from build123d import *

# Parameters (mm, degrees)
SKETCH1_W            = 145.4
SKETCH1_H            = 52.4
BOSS_EXTRUDE1_DEPTH  = 27.2
SKETCH2_W            = 140.4
SKETCH2_H            = 47.4
CUT_EXTRUDE1_DEPTH   = 25.2
SKETCH3_W            = 46.4
SKETCH3_H            = 25.2
CUT_EXTRUDE2_DEPTH   = 25.2
SKETCH8_W            = 2.5
SKETCH8_H            = 52.4
CUT_EXTRUDE5_DEPTH   = 43
SKETCH9_W            = 44.4
SKETCH9_H            = 17.2
CUT_EXTRUDE6_DEPTH   = 43
SKETCH11_W           = 132.9
SKETCH11_H           = 16.2
CUT_EXTRUDE7_DEPTH   = 59
SKETCH12_W           = 130.4
SKETCH12_H           = 42.4
CUT_EXTRUDE8_DEPTH   = 10
SKETCH16_W           = 12
SKETCH16_H           = 2.5
BOSS_EXTRUDE4_DEPTH  = 8
SKETCH18_W           = 12
SKETCH18_H           = 2.5
BOSS_EXTRUDE6_DEPTH  = 8
SKETCH24_W           = 10
SKETCH24_H           = 5
BOSS_EXTRUDE12_DEPTH = 6.2
SKETCH25_W           = 10
SKETCH25_H           = 5
BOSS_EXTRUDE13_DEPTH = 6.2
SKETCH26_W           = 10
SKETCH26_H           = 5
BOSS_EXTRUDE14_DEPTH = 9.7
SKETCH27_W           = 10
SKETCH27_H           = 9
BOSS_EXTRUDE15_DEPTH = 5
SKETCH28_W           = 10
SKETCH28_H           = 2
BOSS_EXTRUDE16_DEPTH = 42.4
SKETCH29_W           = 10
SKETCH29_H           = 2
BOSS_EXTRUDE17_DEPTH = 42.4
SKETCH30_W           = 12
SKETCH30_H           = 4
BOSS_EXTRUDE18_DEPTH = 10
SKETCH35_W           = 10
SKETCH35_H           = 6
BOSS_EXTRUDE22_DEPTH = 9
SKETCH36_W           = 10
SKETCH36_H           = 6
BOSS_EXTRUDE23_DEPTH = 9
SKETCH37_R           = 1.5
CUT_EXTRUDE10_DEPTH  = 9
SKETCH38_W           = 10
SKETCH38_H           = 2
CUT_EXTRUDE11_DEPTH  = 9
SKETCH39_W           = 10
SKETCH39_H           = 2
CUT_EXTRUDE12_DEPTH  = 9
SKETCH40_W           = 10
SKETCH40_H           = 2
CUT_EXTRUDE13_DEPTH  = 9
FILLET1_R            = 1


with BuildPart() as part:
    # Sketch1 → Boss-Extrude1 (new body)
    with BuildSketch(Plane(origin=(0, 0, 0), x_dir=(1, 0, 0), z_dir=(0, 1, 0))):
        Rectangle(SKETCH1_W, SKETCH1_H)
    extrude(amount=BOSS_EXTRUDE1_DEPTH)

    # Sketch2 → Cut-Extrude1 (cut)
    with BuildSketch(Plane(origin=(0, 27.2, 0), x_dir=(1, 0, 0), z_dir=(0, 1, 0))):
        Rectangle(SKETCH2_W, SKETCH2_H)
    extrude(amount=-CUT_EXTRUDE1_DEPTH, mode=Mode.SUBTRACT)

    # Sketch3 → Cut-Extrude2 (cut)
    with BuildSketch(Plane.ZY.offset(-70.2)):
        with Locations((0.5, 14.6)):
            Rectangle(SKETCH3_W, SKETCH3_H)
    extrude(amount=-CUT_EXTRUDE2_DEPTH, mode=Mode.SUBTRACT)

    # Sketch8 → Cut-Extrude5 (cut)
    with BuildSketch(Plane(origin=(0, 27.2, 0), x_dir=(1, 0, 0), z_dir=(0, 1, 0))):
        with Locations((71.45, 0)):
            Rectangle(SKETCH8_W, SKETCH8_H)
    extrude(amount=-CUT_EXTRUDE5_DEPTH, mode=Mode.SUBTRACT)

    # Sketch9 → Cut-Extrude6 (cut)
    with BuildSketch(Plane.ZY.offset(72.7)):
        with Locations((0, 13.6)):
            Rectangle(SKETCH9_W, SKETCH9_H)
    extrude(amount=-CUT_EXTRUDE6_DEPTH, mode=Mode.SUBTRACT)

    # Sketch11 → Cut-Extrude7 (cut)
    with BuildSketch(Plane(origin=(0, 0, -26.2), x_dir=(-1, 0, 0), z_dir=(0, 0, -1))):
        with Locations((1.25, 13.1)):
            Rectangle(SKETCH11_W, SKETCH11_H)
    extrude(amount=-CUT_EXTRUDE7_DEPTH, mode=Mode.SUBTRACT)

    # Sketch12 → Cut-Extrude8 (cut)
    with BuildSketch(Plane(origin=(0, 0, 0), x_dir=(-1, 0, 0), z_dir=(0, -1, 0))):
        Rectangle(SKETCH12_W, SKETCH12_H)
    extrude(amount=-CUT_EXTRUDE8_DEPTH, mode=Mode.SUBTRACT)

    # Sketch16 → Boss-Extrude4 (add)
    with BuildSketch(Plane(origin=(0, 0, -26.2), x_dir=(-1, 0, 0), z_dir=(0, 0, -1))):
        with Locations((-64.2, 25.95)):
            Rectangle(SKETCH16_W, SKETCH16_H)
    extrude(amount=BOSS_EXTRUDE4_DEPTH)

    # Sketch18 → Boss-Extrude6 (add)
    with BuildSketch(Plane.XY.offset(26.2)):
        with Locations((64.2, 25.95)):
            Rectangle(SKETCH18_W, SKETCH18_H)
    extrude(amount=BOSS_EXTRUDE6_DEPTH)

    # Sketch24 → Boss-Extrude12 (add)
    with BuildSketch(Plane.XY.offset(26.2)):
        with Locations((-40.7, 2.5)):
            Rectangle(SKETCH24_W, SKETCH24_H)
        with Locations((32.2, 2.5)):
            Rectangle(SKETCH24_W, SKETCH24_H)
    extrude(amount=BOSS_EXTRUDE12_DEPTH)

    # Sketch25 → Boss-Extrude13 (add)
    with BuildSketch(Plane(origin=(0, 0, -26.2), x_dir=(-1, 0, 0), z_dir=(0, 0, -1))):
        with Locations((40.7, 2.5)):
            Rectangle(SKETCH25_W, SKETCH25_H)
        with Locations((-32.2, 2.5)):
            Rectangle(SKETCH25_W, SKETCH25_H)
    extrude(amount=BOSS_EXTRUDE13_DEPTH)

    # Sketch26 → Boss-Extrude14 (add)
    with BuildSketch(Plane(origin=(0, 0, 0), x_dir=(-1, 0, 0), z_dir=(0, -1, 0))):
        with Locations((40.7, 29.9)):
            Rectangle(SKETCH26_W, SKETCH26_H)
        with Locations((40.7, -29.9)):
            Rectangle(SKETCH26_W, SKETCH26_H)
        with Locations((-32.2, -29.9)):
            Rectangle(SKETCH26_W, SKETCH26_H)
        with Locations((-32.2, 29.9)):
            Rectangle(SKETCH26_W, SKETCH26_H)
    extrude(amount=BOSS_EXTRUDE14_DEPTH)

    # Sketch27 → Boss-Extrude15 (add)
    with BuildSketch(Plane(origin=(0, -9.7, 0), x_dir=(-1, 0, 0), z_dir=(0, -1, 0))):
        with Locations((40.7, -27.9)):
            Rectangle(SKETCH27_W, SKETCH27_H)
        with Locations((-32.2, -27.9)):
            Rectangle(SKETCH27_W, SKETCH27_H)
        with Locations((40.7, 27.9)):
            Rectangle(SKETCH27_W, SKETCH27_H)
        with Locations((-32.2, 27.9)):
            Rectangle(SKETCH27_W, SKETCH27_H)
    extrude(amount=BOSS_EXTRUDE15_DEPTH)

    # Sketch28 → Boss-Extrude16 (add)
    with BuildSketch(Plane.XY.offset(-21.2)):
        with Locations((-40.62922207, 1)):
            Rectangle(SKETCH28_W, SKETCH28_H)
    extrude(amount=BOSS_EXTRUDE16_DEPTH)

    # Sketch29 → Boss-Extrude17 (add)
    with BuildSketch(Plane.XY.offset(-21.2)):
        with Locations((31.742427041, 1)):
            Rectangle(SKETCH29_W, SKETCH29_H)
    extrude(amount=BOSS_EXTRUDE17_DEPTH)

    # Sketch30 → Boss-Extrude18 (add)
    with BuildSketch(Plane(origin=(0, 24.7, 0), x_dir=(-1, 0, 0), z_dir=(0, -1, 0))):
        with Locations((-64.2, -32.2)):
            Rectangle(SKETCH30_W, SKETCH30_H)
        with Locations((-64.2, 32.2)):
            Rectangle(SKETCH30_W, SKETCH30_H)
    extrude(amount=BOSS_EXTRUDE18_DEPTH)

    # Sketch35 → Boss-Extrude22 (add)
    with BuildSketch(Plane(origin=(0, 0, -26.2), x_dir=(-1, 0, 0), z_dir=(0, 0, -1))):
        with Locations((-22.214363523, 24.2)):
            Rectangle(SKETCH35_W, SKETCH35_H)
        with Locations((26.494707746, 24.2)):
            Rectangle(SKETCH35_W, SKETCH35_H)
    extrude(amount=BOSS_EXTRUDE22_DEPTH)

    # Sketch36 → Boss-Extrude23 (add)
    with BuildSketch(Plane.XY.offset(26.2)):
        with Locations((-26.49, 24.2)):
            Rectangle(SKETCH36_W, SKETCH36_H)
        with Locations((22.21, 24.2)):
            Rectangle(SKETCH36_W, SKETCH36_H)
    extrude(amount=BOSS_EXTRUDE23_DEPTH)

    # Sketch37 → Cut-Extrude10 (cut)
    with BuildSketch(Plane.XZ.offset(-21.2)):
        with Locations(Location((-26.49, 31.2, 0), (0, 0, 270))):
            Circle(SKETCH37_R)
        with Locations(Location((22.21, 31.2, 0), (0, 0, 270))):
            Circle(SKETCH37_R)
        with Locations(Location((-26.49, -31.2, 0), (0, 0, 270))):
            Circle(SKETCH37_R)
        with Locations(Location((22.214363523, -31.2, 0), (0, 0, 270))):
            Circle(SKETCH37_R)
    extrude(amount=-CUT_EXTRUDE10_DEPTH, mode=Mode.SUBTRACT)

    # Sketch38 → Cut-Extrude11 (cut)
    with BuildSketch(Plane.XY.offset(35.2)):
        with Locations((-26.49, 22.2)):
            Rectangle(SKETCH38_W, SKETCH38_H)
    extrude(amount=-CUT_EXTRUDE11_DEPTH, mode=Mode.SUBTRACT)

    # Sketch39 → Cut-Extrude12 (cut)
    with BuildSketch(Plane.XY.offset(35.2)):
        with Locations((22.21, 22.2)):
            Rectangle(SKETCH39_W, SKETCH39_H)
    extrude(amount=-CUT_EXTRUDE12_DEPTH, mode=Mode.SUBTRACT)

    # Sketch40 → Cut-Extrude13 (cut)
    with BuildSketch(Plane(origin=(0, 0, -35.2), x_dir=(-1, 0, 0), z_dir=(0, 0, -1))):
        with Locations((-22.214363523, 22.2)):
            Rectangle(SKETCH40_W, SKETCH40_H)
        with Locations((26.494707746, 22.2)):
            Rectangle(SKETCH40_W, SKETCH40_H)
    extrude(amount=-CUT_EXTRUDE13_DEPTH, mode=Mode.SUBTRACT)

    # Fillet1
    fillet1_edges = [part.edges().sort_by_distance(p)[0] for p in [
        (27.214363523, 25.2, -35.2),
        (-21.494707746, 25.2, -35.2),
        (-31.49, 25.2, 35.2),
        (17.21, 25.2, 35.2),
        (-21.49, 25.2, 35.2),
        (27.21, 25.2, 35.2),
        (-31.494707746, 25.2, -35.2),
        (17.214363523, 25.2, -35.2),
    ]]
    fillet(fillet1_edges, radius=FILLET1_R)


solid = part.part
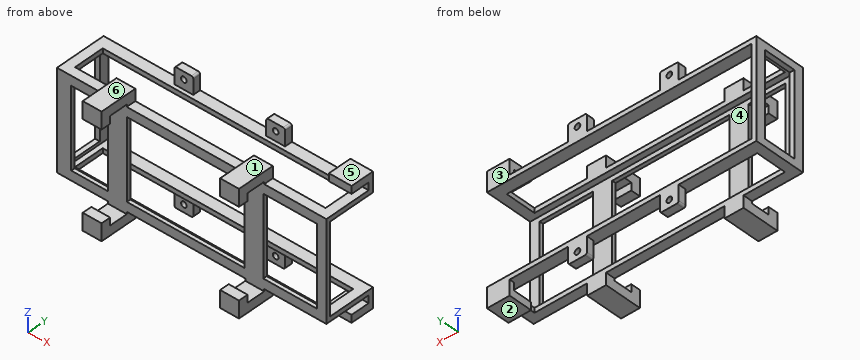
Check sheet for the modelled part. Datum: model origin and axes. Units: mm. Face numbers are marked on the shaded views. A direction names the side the tool comes from. Round coordinates to 2 decimals unless told otherwise and drop trailing zeros. Loops run counter-clockwise (first coordinate to the right, second up) from the corner with the lowest first, then second, coordinate; pieces in that order, holes last. Notation, with made-up numbers: (59, 12) - (116, 12) arc R14 ccw to (116, 28) - close; hole circle Ø7 at (49.5, -38.5). An arc over 180 degrees is marked (long way). Answer as CSV lines item,"result". Start each with the question number.
Item 1: Section check B-B (y = 10.5). Record the boundary of the cut face in (x, z), and give its area (3 significant figures).
Item 2: Scan lines: line 1 (X direction, y = 1, z = 15.5); line 2 (X direction, y = 25, z = 31); line 3 (Z direction, x = 22, y = 24). Record each from-to range of solid material in increasing order. Write a range as [from, to].
Item 3: Depth check by flat-ended pin: P1, Ø3, axis at x = -41.5, y = -3, coming from the -Z side; P2, Ø1, axis at y = 20, z = 6.5, coming from the -X side (1 decimal); P3, Ø1.2, axis at y = 25, z = -32, coming from the -X side; P4, Ø2, axis at x = -71, y = 16.5, coming from the +Z side. Enter the tip coordinate at first touch or a pass-through.
Item 4: Set-up check for the marked faces 5 and 6: record each of +Z, -Z, +X, -X, +Y, -Y from which the full face is reachable in a straight line by a thin tool's end or side.
Item 5: Section check A-A (x = 33). Record the boundary of the cut face in (y, z).
Item 6: Section check C-C (x = -63.5). Record the boundary of the cut face in (y, z), and give its area (3 significant figures).
Item 7: Release check for a two-part mould opening along Z. For the marked faces 1, 2, 3 and 4 record: +Z half, -Z half, draft (parallel to the pull), parting line (faces both ways), or undercut.
Item 8: Section check D-D (z = -11). Record the boundary of the cut face in (x, y), and give its area (3 significant figures).
Report:
1,outline,"(-72.7, -26.2) - (-67.7, -26.2) - (-67.7, -23.7) - (-70.2, -23.7) - (-70.2, -22.2) - (-72.7, -22.2) - close; (-72.7, 22.2) - (-70.2, 22.2) - (-70.2, 23.7) - (-67.7, 23.7) - (-67.7, 26.2) - (-72.7, 26.2) - close; (65.2, -26.2) - (70.2, -26.2) - (70.2, -23.7) - (65.2, -23.7) - close; (65.2, 23.7) - (70.2, 23.7) - (70.2, 26.2) - (65.2, 26.2) - close"
1,area,"57.5 mm2"
2,line 1,"x = [-72.7, -65.2], [-45.63, -35.63], [26.74, 36.74], [65.2, 70.2]"
2,line 2,"x = [-31.49, -27.98], [-25, -21.49], [17.21, 20.72], [23.7, 27.21], [58.2, 70.2]"
2,line 3,"z = [-35.2, -32.68], [-29.72, -23.7], [23.7, 29.71], [32.69, 35.2]"
3,P1,"stops at z = -32.4"
3,P2,"passes through"
3,P3,"stops at x = -31.49"
3,P4,"stops at z = 26.2"
4,face 5,"+Z, +X, +Y, -Y"
4,face 6,"+Z, +X, -X, +Y, -Y"
5,outline,"(-14.7, -32.4) - (5, -32.4) - (5, -23.7) - (2, -23.7) - (2, 23.7) - (5, 23.7) - (5, 32.4) - (-14.7, 32.4) - (-14.7, 23.4) - (-9.7, 23.4) - (-9.7, 27.4) - (0, 27.4) - (0, -27.4) - (-9.7, -27.4) - (-9.7, -23.4) - (-14.7, -23.4) - close; (21.2, -26.2) - (27.2, -26.2) - (27.2, -23.7) - (21.2, -23.7) - close; (21.2, 23.7) - (27.2, 23.7) - (27.2, 26.2) - (21.2, 26.2) - close"
6,outline,"(0, -26.2) - (5, -26.2) - (5, -23.7) - (2, -23.7) - (2, -21.2) - (0, -21.2) - close; (0, 21.2) - (2, 21.2) - (2, 23.7) - (5, 23.7) - (5, 26.2) - (0, 26.2) - close; (21.2, -26.2) - (27.2, -26.2) - (27.2, -23.7) - (21.2, -23.7) - close; (21.2, 23.7) - (27.2, 23.7) - (27.2, 26.2) - (21.2, 26.2) - close"
6,area,"65.0 mm2"
7,face 1,"+Z half"
7,face 2,"-Z half"
7,face 3,"draft"
7,face 4,"undercut"
8,outline,"(-72.7, 0) - (-65.2, 0) - (-65.2, 2) - (-70.2, 2) - (-70.2, 5) - (-72.7, 5) - close; (-72.7, 22.2) - (-70.2, 22.2) - (-70.2, 27.2) - (-72.7, 27.2) - close; (-45.63, 0) - (-35.63, 0) - (-35.63, 2) - (-45.63, 2) - close; (26.74, 0) - (36.74, 0) - (36.74, 2) - (26.74, 2) - close; (65.2, 0) - (70.2, 0) - (70.2, 2) - (65.2, 2) - close"
8,area,"85.0 mm2"
